Input: part model. Units: mm. Frame: model coordinates. A direction names the side the tool comes from. Round coordinates to 2 decimals unless told otherwise and drop trailing zeros. Loops run counter-clockwise (first coordinate to the right, second up) from the corner with the lowest first, then second, coordinate; pieces in that order, holes last. Notation, with made-up numbers: M -17.75,13.25 L 27.25,13.25 A28 ccw 27.25,47.25 Z; hole C 75.5,-23.75 d3. An arc over 180 degrees is marked long. Return JSON: item names as keys, results as strings. Group by question number.
1) Access query for faces 3 (the face through (35, 100, -27)), 4 (the face through (-29, 100, -11)), 5 (the face through (61.2, 92.58, -32.53)), 6 (the face through (12, 103, -26)). Directions: +Z, -Z, +X, -X, +Y, -Y. A direction counts if a zero-diameter tool reaches every point of the face in a straight line with its end or side. Return the directions, or none.
2) Section C-C (y = 100). Count the separate pieces of the cut face and the enclosed holes in it, plus the area to 3 significant figures.
3) Contact query for flat-ended pins moving along their axis: P1, Ø6, axis at x = 28.5, y = 100, coming from the +Z side; P2, Ø8, axis at y = 109, z = -19.5, coming from the -X side; P3, Ø3, axis at x = 44, y = 101, coming from the -Z side. Output: stop coordinate, or through.
4) Section B-B (z = -3.5). Output: boundary loops of the cut face in (x, y).
5) Material intervals for line 1 (X direction, y = 107.5, z = -32.8); line 2 (Y direction, x = -57, z = -32); line 3 (X direction, y = 99.45, z = -28), sorted ascending. Write a range as from..to.
6) Mould query, pull axis X, two halves, no side actions, for faces 1 (the face through (-47, 100, -30)), 2 (the face through (59.5, 108, -33)). Classes: +X half, -X half, draft (parallel to the pull), parting line (faces both ways), or undercut.
7) Section D-D (x = -51.5). Output: boundary loops of the cut face in (y, z), plus the area to 3 significant figures.
8) Section A-A (x = 63). Output: boundary loops of the cut face in (y, z).
from build123d import *

# Parameters (mm, degrees)
PAD_DEPTH            = 110
SKETCH002_R          = 3.45
POCKET001_DEPTH      = 11
SKETCH004_R          = 2.1
POCKET003_DEPTH      = 7.001
POCKET003_DEPTH_BACK = 7.001
SKETCH005_W          = 7
SKETCH005_H          = 8
POCKET004_DEPTH      = 7.001
POCKET004_DEPTH_BACK = 7.001
PAD001_DEPTH         = 8
SKETCH003_R          = 19
POCKET_DEPTH         = 9
SKETCH001_R          = 21
POCKET005_DEPTH      = 4.6
SKETCH007_W          = 27
SKETCH007_H          = 25
SKETCH007_R          = 1.8
PAD002_DEPTH         = 5
LINEARPATTERN_COUNT  = 2
LINEARPATTERN_PITCH  = 120
CHAMFER002_SIZE      = 1
CHAMFER003_SIZE      = 1


with BuildPart() as part:
    # Sketch → Pad (new body)
    with BuildSketch(Plane.YZ.offset(-42)):
        Polygon((-7, 0), (7, 0), (7, -10), (3, -17), (3, -35), (-3, -35), (-3, -17), (-7, -10), align=None)
    extrude(amount=PAD_DEPTH)

    # Sketch002 → Pocket001 (cut)
    with BuildSketch(Plane.XY):
        with Locations((-28.5, 0)):
            Circle(SKETCH002_R)
        with Locations((28.5, 0)):
            Circle(SKETCH002_R)
    extrude(amount=-POCKET001_DEPTH, mode=Mode.SUBTRACT)

    # Sketch004 → Pocket003 (cut, two sides)
    with BuildSketch(Plane.XZ) as pocket003_sk:
        with Locations((-10, -28)):
            Circle(SKETCH004_R)
        with Locations((10, -28)):
            Circle(SKETCH004_R)
    extrude(amount=-POCKET003_DEPTH, mode=Mode.SUBTRACT)
    extrude(pocket003_sk.sketch, amount=POCKET003_DEPTH_BACK, mode=Mode.SUBTRACT)

    # Sketch005 → Pocket004 (cut, two sides)
    with BuildSketch(Plane.XZ) as pocket004_sk:
        with Locations((35.5, -31)):
            Rectangle(SKETCH005_W, SKETCH005_H)
        with Locations((45.5, -31)):
            Rectangle(SKETCH005_W, SKETCH005_H)
    extrude(amount=-POCKET004_DEPTH, mode=Mode.SUBTRACT)
    extrude(pocket004_sk.sketch, amount=POCKET004_DEPTH_BACK, mode=Mode.SUBTRACT)

    # Sketch006 → Pad001 (join, symmetric)
    with BuildSketch(Plane.XZ):
        with BuildLine():
            Line((-24, 0), (24, -5.7e-05))
            ThreePointArc((-24, 0), (-2.8e-05, -24), (24, -5.7e-05))
        make_face()
    extrude(amount=PAD001_DEPTH, both=True)

    # Sketch003 → Pocket (cut, symmetric)
    with BuildSketch(Plane.XZ):
        Circle(SKETCH003_R)
    extrude(amount=POCKET_DEPTH, both=True, mode=Mode.SUBTRACT)

    # Sketch001 → Pocket005 (cut, symmetric)
    with BuildSketch(Plane.XZ):
        Circle(SKETCH001_R)
    extrude(amount=POCKET005_DEPTH, both=True, mode=Mode.SUBTRACT)

    # Sketch007 → Pad002 (join)
    with BuildSketch(Plane(origin=(-123, -11.5, -35), x_dir=(1, 0, 0), z_dir=(0, 0, 1))):
        with Locations((76, 11.5)):
            Rectangle(SKETCH007_W, SKETCH007_H)
        with Locations((66, 19)):
            Circle(SKETCH007_R, mode=Mode.SUBTRACT)
        with Locations((86, 19)):
            Circle(SKETCH007_R, mode=Mode.SUBTRACT)
        with Locations((86, 4)):
            Circle(SKETCH007_R, mode=Mode.SUBTRACT)
        with Locations((66, 4)):
            Circle(SKETCH007_R, mode=Mode.SUBTRACT)
    pad002 = extrude(amount=PAD002_DEPTH)

    # LinearPattern: Pad002 ×2
    with Locations(*[(i * LINEARPATTERN_PITCH, 0, 0) for i in range(1, LINEARPATTERN_COUNT)]):
        add(pad002)

    # Chamfer002
    chamfer002_edges = [part.edges().sort_by_distance(p)[0] for p in [
        (73, -12.5, -30),
        (73, 12.5, -30),
        (86.5, 0, -30),
        (59.5, -7.75, -30),
        (59.5, 7.75, -30),
    ]]
    chamfer(chamfer002_edges, length=CHAMFER002_SIZE)

    # Chamfer003
    chamfer003_edges = [part.edges().sort_by_distance(p)[0] for p in [
        (-47, -12.5, -30),
        (-33.5, -7.75, -30),
        (-60.5, 0, -30),
        (-47, 12.5, -30),
        (-60.5, -12.5, -32.5),
        (-33.5, -12.5, -32.5),
        (-60.5, 12.5, -32.5),
        (-33.5, 7.75, -30),
    ]]
    chamfer(chamfer003_edges, length=CHAMFER003_SIZE)


with BuildPart() as part_1:
    # Body001 placement: moved
    add(part.part.moved(Location((0, 100, 0))))


solid = part_1.part
Returned:
{
 "1": {"face 3": "-Z, +Y, -Y", "face 4": "+Z", "face 5": "-Z", "face 6": "+Y"},
 "2": {"separate pieces": "1", "enclosed holes": "2", "area": "3,050 mm^2"},
 "3": {"P1": "stops at z = -11", "P2": "stops at x = -18.22", "P3": "stops at z = -27"},
 "4": {"outline": "M -42,93 L -23.74,93 L -23.74,92 L -18.67,92 L -18.67,95.4 L -20.71,95.4 L -20.71,104.6 L -18.67,104.6 L -18.67,108 L -23.74,108 L -23.74,107 L -42,107 Z; M 18.67,92 L 23.74,92 L 23.74,93 L 68,93 L 68,107 L 23.74,107 L 23.74,108 L 18.67,108 L 18.67,104.6 L 20.71,104.6 L 20.71,95.4 L 18.67,95.4 Z; hole C -28.5,100 d6.9; hole C 28.5,100 d6.9"},
 "5": {"line 1": "x = -60.5..-58.8, -55.2..-38.8, -35.2..-33.5, 59.5..61.2, 64.8..81.2, 84.8..86.5", "line 2": "y = 87.5..90.7, 94.3..105.7, 109.3..112.5", "line 3": "x = -42..-12.1, -7.9..7.9, 12.1..32, 39..42, 49..68"},
 "6": {"face 1": "draft", "face 2": "undercut"},
 "7": {"outline": "M 87.5,-35 L 112.5,-35 L 112.5,-31 L 111.5,-30 L 88.5,-30 L 87.5,-31 Z", "area": "124 mm^2"},
 "8": {"outline": "M 87.5,-35 L 90.7,-35 L 90.7,-30 L 88.5,-30 L 87.5,-31 Z; M 93,-10 L 97,-17 L 97,-30 L 94.3,-30 L 94.3,-35 L 105.7,-35 L 105.7,-30 L 103,-30 L 103,-17 L 107,-10 L 107,0 L 93,0 Z; M 109.3,-35 L 112.5,-35 L 112.5,-31 L 111.5,-30 L 109.3,-30 Z"}
}
